from build123d import *

# Parameters (mm, degrees)
F0_W     = 304.8
F0_H     = 304.8
F1_DEPTH = 152.4
F3_DEPTH = 152.4
F5_DEPTH = 152.4


with BuildPart() as f1:
    # F0 (on Top) → F1 (new body, symmetric)
    with BuildSketch(Plane.XY):
        Rectangle(F0_W, F0_H)
    extrude(amount=F1_DEPTH, both=True)

    # F2 (on Right) → F3 (cut, symmetric)
    with BuildSketch(Plane.YZ):
        with BuildLine():
            Line((-152.4, 152.4), (0, 152.4))
            ThreePointArc((0, 152.4), (-260.163073, 260.163073), (-152.4, 0))
            Line((-152.4, 0), (-152.4, 152.4))
        make_face()
        with BuildLine():
            ThreePointArc((-152.4, 0), (-44.636927, 44.636927), (0, 152.4))
            Line((0, 152.4), (-152.4, 152.4))
            Line((-152.4, 152.4), (-152.4, 0))
        make_face()
        with BuildLine():
            Line((152.4, 152.4), (0, 152.4))
            ThreePointArc((0, 152.4), (44.636927, 44.636927), (152.4, 0))
            Line((152.4, 0), (152.4, 152.4))
        make_face()
    extrude(amount=F3_DEPTH, both=True, mode=Mode.SUBTRACT)

    # F4 (on Front) → F5 (cut, symmetric)
    with BuildSketch(Plane.XZ):
        with BuildLine():
            Line((152.4, 152.4), (0, 152.4))
            ThreePointArc((0, 152.4), (44.636927, 44.636927), (152.4, 0))
            Line((152.4, 0), (152.4, 152.4))
        make_face()
        with BuildLine():
            ThreePointArc((-152.4, 0), (-44.636927, 44.636927), (0, 152.4))
            Line((0, 152.4), (-152.4, 152.4))
            Line((-152.4, 152.4), (-152.4, 0))
        make_face()
    extrude(amount=F5_DEPTH, both=True, mode=Mode.SUBTRACT)


solid = f1.part
Verification items for the finished model (mm, model axes). Coordinates: 2 decimals unless noted, no trailing zeros. Order: outer loops, then holes, each group sorted by start corner. A loop starts at its lowest first (then second) coordinate and runs counter-clockwise, first axis right, second up. Notation, with made-up numbers: (-4.5, -9.75) -> (33.5, -9.75) arc R20 ccw to (33.5, 8.25) -> close; hole circle Ø6 at (76.25, -21). An arc over 180 degrees is marked (long way). Put each result on its own line as item: value. Start each with the question number.
1. Cross-section at B-B, the plane x = -95.5. Record the boundary of the cut face in (y, z).
2. Material ranges on L1, parallel to Y at x = -67, z = 13; L2, parallel to Z at x = 13.5, y = 14; L3, parallel to Z at x = 132.5, y = 14, recorded low to high. Write a range as [from, to].
3. Cross-section at A-A, the plane y = -66. Record the boundary of the cut face in (x, z).
4. Go/stop test with a flat-tipped pin: pin 1 Ø4 at (x, z) = (-21, 79.5) entering from +Y. Record where the tip stops, or that it passes through.
5. Cross-section at C-C, the plane z = 66. Record the boundary of the cut face in (x, y).
Computed:
1. outline: (-152.4, -152.4) -> (152.4, -152.4) -> (152.4, 0) arc R152.4 cw to (95.5, 11.02) -> (-95.5, 11.02) arc R152.4 cw to (-152.4, 0) -> close
2. L1: [-90.81, 90.81]
2. L2: [-152.4, 88.59]
2. L3: [-152.4, 1.3]
3. outline: (-152.4, -152.4) -> (152.4, -152.4) -> (152.4, 0) arc R152.4 cw to (66, 26.86) -> (-66, 26.86) arc R152.4 cw to (-152.4, 0) -> close
4. pin 1: through
5. outline: (-26.86, -26.86) -> (26.86, -26.86) -> (26.86, 26.86) -> (-26.86, 26.86) -> close
